from build123d import *

# Parameters (mm, degrees)
CUT_EXTRUDE1_DEPTH = 2.032
CUT_EXTRUDE1_TAPER = 8


with BuildPart() as part:
    # Sketch1 → Base-Revolve (revolve)
    with BuildSketch(Plane.XY):
        with BuildLine():
            Line((0, 0), (1.5875, 0))
            Line((1.5875, 0), (1.5875, 10.414))
            Line((1.5875, 10.414), (3.81, 10.414))
            Line((3.81, 10.414), (3.81, 11.43))
            Line((3.81, 11.43), (2.9718, 11.43))
            ThreePointArc((2.9718, 11.43), (1.615897215, 12.369193484), (0, 12.7))
            Line((0, 12.7), (0, 0))
        make_face()
    revolve(axis=Axis((0, 0, 0), (0, 1, 0)))

    # Sketch2 → Cut-Extrude1 (cut)
    with BuildSketch(Plane(origin=(0, 12.7, 0), x_dir=(-1, 0, 0), z_dir=(0, 1, 0))):
        Polygon((0.381, 1.397), (-0.381, 1.397), (-0.381, 0.381), (-1.397, 0.381), (-1.397, -0.381), (-0.381, -0.381), (-0.381, -1.397), (0.381, -1.397), (0.381, -0.381), (1.397, -0.381), (1.397, 0.381), (0.381, 0.381), align=None)
    extrude(amount=-CUT_EXTRUDE1_DEPTH, taper=CUT_EXTRUDE1_TAPER, mode=Mode.SUBTRACT)


solid = part.part
The listing builds one solid part. Answer for the finished solid, in the listing's coordinates (mm). A direction names the side the tool comes from. Give positions to 0.01 mm unless a question says otherwise; leave off trailing zeros. Write each loop counter-clockwise with the first axis right and the second up, starting at its lowest first coordinate (ties: lowest second). Pieces come first, ordered by that corner, then holes.
1) Given P1, Ø1, axis at x = 1, z = 0, coming from the -Y side; P2, Ø2, axis at x = -1.5, y = 3, coming from the +Z side; P3, Ø1.5, axis at y = 6.5, z = 3, coming from the -X side, each flat-ended and moving along its own axis, determine where each tip first touches the part or whether it passes through.
2) Section B-B (y = 3.75) is taken. Write down the section's boundary in (x, z) (1 decimal), and give its area (3 significant figures).
3) Section C-C (z = 3.25) is taken. Write down the section's boundary in (x, y).
4) Find the intervals of material crossed by L1, parallel to Y at x = 3.5, z = 0; L2, parallel to Y at x = -0.5, z = 0.75; L3, parallel to X at y = 0.5, z = 0.5, in increasing order.
5) Section A-A (x = -2.75) is taken. Write down the section's boundary in (y, z), and give its area (3 significant figures).
6) A tool of negligible diameter and unlimited length cuts with its end or side. For faces 1 (the face through (-1, 11.43, 3)), 2 (the face through (-0.34, 5.28, 1.55)), 3 (the face through (0, 0, 0)), from which of +Z, -Z, +X, -X, +Y, -Y can it reach the whole face along a straight path? Write none if from no direction.
Response:
1. P1: stops at y = 0
1. P2: stops at z = 1.51
1. P3: passes through
2. outline: circle Ø3.2 at (0, 0)
2. area: 7.92 mm2
3. outline: (-1.99, 10.41) - (1.99, 10.41) - (1.99, 11.43) - (-1.99, 11.43) - close
4. L1: y = 10.41 to 11.43
4. L2: y = 0 to 12.6
4. L3: x = -1.51 to 1.51
5. outline: (10.41, -2.64) - (11.43, -2.64) - (11.43, -1.13) arc R3.06 ccw to (11.43, 1.13) - (11.43, 2.64) - (10.41, 2.64) - close
5. area: 5.68 mm2
6. face 1: +Y
6. face 2: -Y
6. face 3: +Z, -Z, +X, -X, -Y
